Autodesk Inventor part; units mm, degrees
ref_plane "Work Plane1" through (-16.7887, 0, 0) normal (0, -0.866, -0.5) x (1, 0, 0)
ref_plane "YZ Plane" through (0, 0, 0) normal (1, 0, 0) x (0, 1, 0)
ref_plane "XZ Plane" through (0, 0, 0) normal (0, 1, 0) x (-1, 0, 0)
sketch "Sketch1" plane through (0, 0, 0) normal (1, 0, 0) x (0, 1, 0)
  line L0 (-8.2416, 0) -> (-4.1208, 7.1374)
  line L1 (-4.1208, 7.1374) -> (4.1208, 7.1374)
  line L2 (4.1208, 7.1374) -> (8.2416, 0)
  line L3 (8.2416, 0) -> (4.1208, -7.1374)
  line L4 (4.1208, -7.1374) -> (-4.1208, -7.1374)
  line L5 (-4.1208, -7.1374) -> (-8.2416, 0)
  point P0 (0, 0)
  point P1 (0, 0)
  dimension "d0" = 16.4831
extrude "Body" add sketch "Sketch1" along normal blind 5.7658
sketch "Sketch2" plane through (0, 0, 0) normal (0, 0, 1) x (1, 0, 0)
  line L0 (0, 4.1208) -> (0, 8.2416)
  line L1 (0, 8.2416) -> (5.7658, 8.2416)
  line L2 (5.7658, 4.1208) -> (5.7658, 8.2416)
  line L3 (-1.1532, 0) -> (6.919, 0)
  line L4 (0.6375, 8.2416) -> (0, 7.1374)
  line L5 (5.1283, 8.2416) -> (5.7658, 7.1374)
  dimension "d3" = 30
  dimension "d4" = 30
  dimension "d5" = 14.2748
  dimension "d6" = 14.2748
revolve "Chamfer1" cut sketch "Sketch2" angle 360 about axis through (-10, 0, 0) along (1, 0, 0)
sketch "Sketch3" plane through (5.7658, 0, 0) normal (1, 0, 0) x (0, 0, -1)
  arc A0 (-3.5687, -6.1812) -> (3.5687, -6.1812) centre (0, 0) ccw
hole "Thread" at (5.7658, 0, 0) direction (-1, 0, 0) diameter 7.7978 end through all
chamfer "Chamfer2" distance 0.8593 angle 30 1 edges at (5.7658, 0, 3.8989) measured on face at (5.7658, 6.0224, 0.1567)
chamfer "Chamfer3" distance 0.8593 angle 30 1 edges at (0, 0, 3.8989) measured on face at (0, 6.0224, 0.1567)
ref_plane "Work Plane1" through (-16.7887, 0, 0) normal (0, -0.866, -0.5) x (1, 0, 0)
equation "\"d0\" = 1.1547 * SW"
equation "\"d1\" = KOH"
equation "\"d3\" = ANG1"
equation "\"d4\" = ANG2"
equation "\"d5\" = SW0"
equation "\"d6\" = SW01"
equation "\"d8\" = -0.5 * GD1 + 0.5 * NND"
equation "\"d40\" = -0.5 * GD1 + 0.5 * NND"
equation "\"d10\" = -0.5 * GD1 + 0.5 * NND"
equation "\"d41\" = -0.5 * GD1 + 0.5 * NND"
equation "\"ANG1\" = 30deg"
equation "\"ANG2\" = 30deg"
equation "\"NND\" = 9.525"
equation "\"KOH\" = 5.7658"
equation "\"SW\" = 14.2748"
equation "\"SW0\" = SW"
equation "\"SW01\" = SW"
equation "\"THREADDIA\" = 9.525"
equation "\"TOA\" = 30deg"
equation "\"E0\" = 1.155 * SW"
properties part number "AS 2465 - 3/8  UNC" material "Steel, Mild"
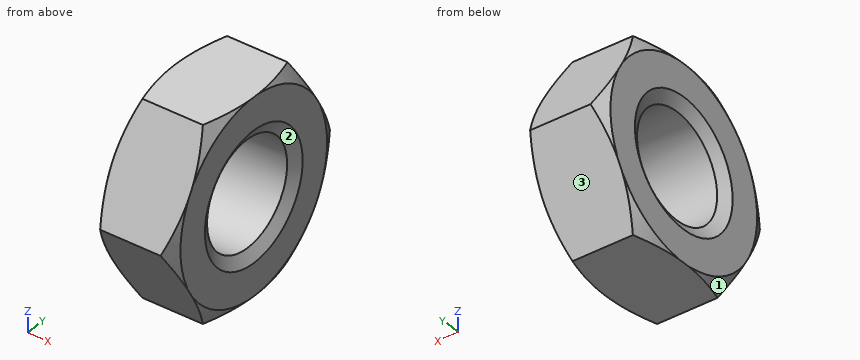
The listing builds one solid part. Answer for the finished solid, in the listing's coordinates (mm). Face numbers are marked on the shaded views. Coordinates: 2 decimals unless noted, no trailing zeros. Order: outer loops, then holes, each group sorted by start corner. A loop starts at its lowest first (then second) coordinate and runs counter-clockwise, first axis right, second up.
Q1. For a pull along Z with two mould halves and no side action, classify the marked faces 1, 2 and 3 as pulls with the +Z half, pulls with the -Z half, needs draft (parallel to the pull), parting line crosses it, or undercut.
Q2. Consider line 1 (Z direction, x = 2.45, y = 0); line 2 (Y direction, x = 4.5, z = 3.5); line 3 (Y direction, x = 5, z = -1). Determine where each line is inside the solid, lowest interval first.
Q3. A cutting plane is placed at A-A, the plane x = 1.65. Write down the section's boundary in (y, z), and give its area (3 significant figures).
Q4. Given P1, Ø5, axis at y = 5, z = -4, coming from the -X side; P2, Ø1.5, axis at x = 3.5, z = -4, coming from the +Y side, each flat-ended and moving along its own axis, determine where each tip first touches the part or whether it passes through.
Answers follow:
1. face 1: parting line crosses it
1. face 2: undercut
1. face 3: pulls with the -Z half
2. line 1: z = -7.14 to -3.9, 3.9 to 7.14
2. line 2: y = -6.22 to -1.72, 1.72 to 6.22
2. line 3: y = -7.66 to -3.77, 3.77 to 7.66
3. outline: (-8.24, 0) - (-4.12, -7.14) - (4.12, -7.14) - (8.24, 0) - (4.12, 7.14) - (-4.12, 7.14) - close; hole circle Ø7.8 at (0, 0)
3. area: 129 mm2
4. P1: stops at x = 0
4. P2: stops at y = 6.37
